Answer from the drawing. Dimensions are ordinates in mm from the lowest x, y and z of the part. Coordinates: 2 decimals unless noted, no trailing zeros. Loops run counter-clockwise (first coordinate to the right, second up) from the corner with the lowest first, then second, coordinate; pieces in that order, holes last. Notation, with made-up numbers: M 40.5,41.5 L 70.5,41.5 A8 ccw 70.5,49.5 Z; hole C -37,72 d1. An arc over 180 degrees is marked long. Put each result on its own line as item: value.
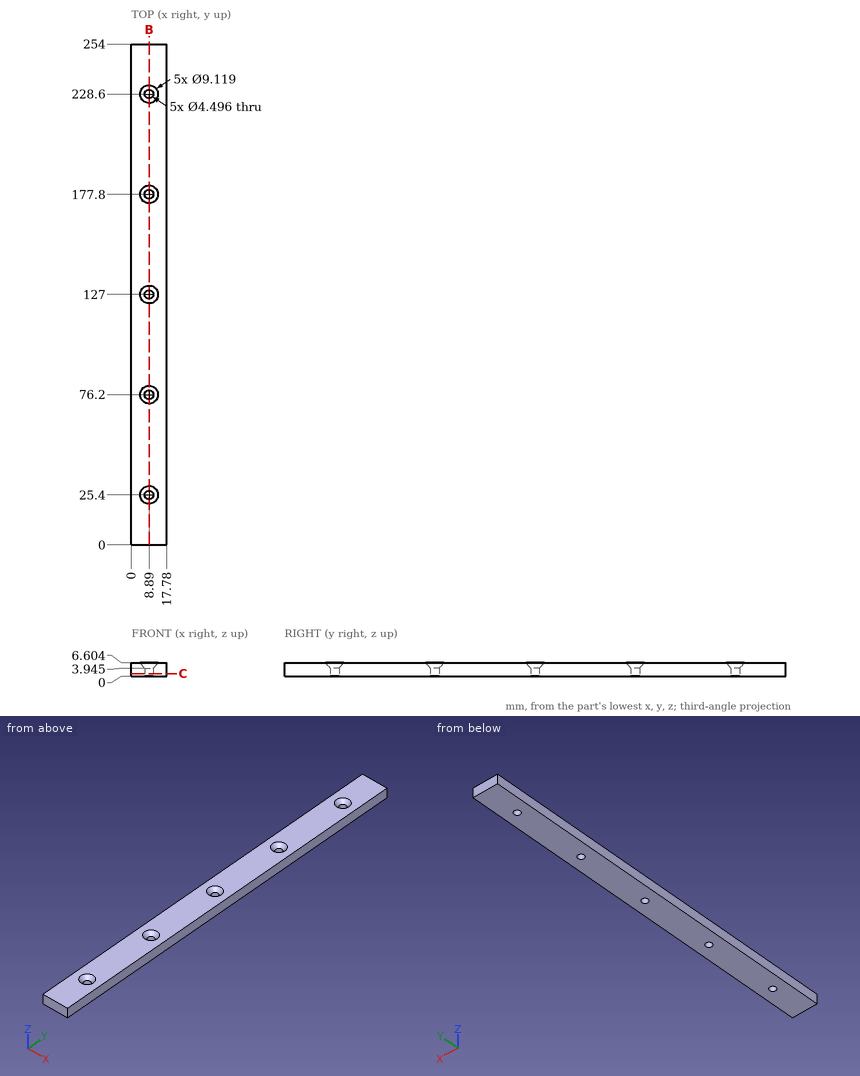
1) Find section C-C, the plane z = 1.25. Write down the section's boundary in (x, y) (1 decimal), plus the area to 3 significant figures.
Answer list:
outline: M 0,0 L 17.8,0 L 17.8,254 L 0,254 Z; hole C 8.9,25.4 d4.5; hole C 8.9,76.2 d4.5; hole C 8.9,127 d4.5; hole C 8.9,177.8 d4.5; hole C 8.9,228.6 d4.5
area: 4,440 mm^2
2) Given pin 1 Ø7 at (x, y) = (8.89, 25.4) entering from +Z (1 decimal); pin 2 Ø6 at (x, y) = (8.89, 127) entering from -Z, each flat-ended and moving along its own axis, determine where each tip first touches the part or whether it passes through.
Answer list:
pin 1: stops at z = 5.4
pin 2: stops at z = 0
3) Find section B-B, the plane x = 8.89. Count the separate pieces of the cut face and the enclosed holes in it, plus the area to 3 significant figures.
Answer list:
separate pieces: 6
enclosed holes: 0
area: 1,500 mm^2
4) Straight lines are drawn through the part: line 1 (Y direction, x = 8.89, z = 2); line 2 (Y direction, x = 7, z = 1) (1 decimal); line 3 (X direction, y = 76.2, z = 3). For each, find the intervals that lie inside material, in ascending order. Write a range as [from, to].
Answer list:
line 1: y = [0, 23.15], [27.65, 73.95], [78.45, 124.75], [129.25, 175.55], [180.05, 226.35], [230.85, 254]
line 2: y = [0, 24.2], [26.6, 75], [77.4, 125.8], [128.2, 176.6], [179, 227.4], [229.8, 254]
line 3: x = [0, 6.64], [11.14, 17.78]
